The model under review builds one solid part; all positions refer to its coordinate system, in mm. A direction names the side the tool comes from. Coordinates: 2 decimals unless noted, no trailing zeros. Loops run counter-clockwise (first coordinate to the right, second up) from the corner with the lowest first, then second, coordinate; pieces in that order, holes last. Notation, with made-up numbers: M 13.25,-31.75 L 57.25,-31.75 A17 ccw 57.25,-21.75 Z; hole C 14.5,30 d11. An arc over 180 degrees is marked long. Return JSON: item names as keys, results as strings.
```python
from build123d import *

# Parameters (mm, degrees)
CROQUIS2_R              = 45
CROQUIS2_R_2            = 41
SALIENTE_EXTRUIR1_DEPTH = 10
CROQUIS3_R              = 45
SALIENTE_EXTRUIR2_DEPTH = 10
CROQUIS4_R              = 45
CROQUIS4_R_2            = 39.9
SALIENTE_EXTRUIR3_DEPTH = 3
CROQUIS5_R              = 2.5
CORTAR_EXTRUIR1_DEPTH   = 10


with BuildPart() as part:
    # Croquis2 → Saliente-Extruir1 (new body)
    with BuildSketch(Plane(origin=(0, 0, 0), x_dir=(0, 0, -1), z_dir=(1, 0, 0))):
        with Locations((-3.334066787, 2.439156595)):
            Circle(CROQUIS2_R)
        with Locations((-3.334066787, 2.439156595)):
            Circle(CROQUIS2_R_2, mode=Mode.SUBTRACT)
    extrude(amount=SALIENTE_EXTRUIR1_DEPTH)

    # Croquis3 → Saliente-Extruir2 (add)
    with BuildSketch(Plane(origin=(0, 0, 0), x_dir=(0, 0, -1), z_dir=(1, 0, 0))):
        with Locations((-3.334066787, 2.439156595)):
            Circle(CROQUIS3_R)
    extrude(amount=-SALIENTE_EXTRUIR2_DEPTH)

    # Croquis4 → Saliente-Extruir3 (add)
    with BuildSketch(Plane(origin=(10, 0, 0), x_dir=(0, 0, -1), z_dir=(1, 0, 0))):
        with Locations((-3.334066787, 2.439156595)):
            Circle(CROQUIS4_R)
        with Locations((-3.334066787, 2.439156595)):
            Circle(CROQUIS4_R_2, mode=Mode.SUBTRACT)
    extrude(amount=-SALIENTE_EXTRUIR3_DEPTH)

    # Croquis5 → Cortar-Extruir1 (cut)
    with BuildSketch(Plane(origin=(0, 0, 0), x_dir=(0, 0, -1), z_dir=(1, 0, 0))):
        with Locations((-3.334066787, 2.439156595)):
            Circle(CROQUIS5_R)
    extrude(amount=-CORTAR_EXTRUIR1_DEPTH, mode=Mode.SUBTRACT)


solid = part.part
```
1. Add section D-D on x = 1.75. Give the boundary of the cut face in (y, z).
Check values:
{"outline": "C 2.44,3.33 d90; hole C 2.44,3.33 d82"}
2. Add section B-B on y = -7. Give the boundary of the cut face in (x, z), plus the area to 3 significant figures.
Check values:
{"outline": "M -10,-40.66 L 10,-40.66 L 10,-35.43 L 7,-35.43 L 7,-36.56 L 0,-36.56 L 0,43.23 L 7,43.23 L 7,42.1 L 10,42.1 L 10,47.33 L -10,47.33 Z", "area": "969 mm²"}
3. Add section C-C on z = 2.5. Give the boundary of the cut face in (x, y), plus the area to 3 significant figures.
Check values:
{"outline": "M -10,-42.55 L 10,-42.55 L 10,-37.45 L 7,-37.45 L 7,-38.55 L 0,-38.55 L 0,0.08 L -10,0.08 Z; M -10,4.8 L 0,4.8 L 0,43.43 L 7,43.43 L 7,42.33 L 10,42.33 L 10,47.43 L -10,47.43 Z", "area": "939 mm²"}
4. Insertion check: pin 1 Ø1.5 at (x, z) = (-3, -17) entering from +Y; pin 2 Ø5 at (y, z) = (30.5, 5) entering from +X; pin 3 Ø10 at (x, z) = (-5, -12) entering from +Y; pin 4 Ø8 at (y, z) = (2.44, 3.33) entering from -X. Each pin has a flat end and moves straight along its axis. Give the tip position at first contact, or say it passes through.
Check values:
{"pin 1": "y = 42.95", "pin 2": "x = 0", "pin 3": "y = 46.24", "pin 4": "x = -10"}
5. The part is to be moulded in two halves that separate along X. For faces 1 (the face through (0.14, -41.49, 13.09)), 2 (the face through (3.451, -37.586, 12.222)), 3 (the face through (-10, 3, -6)), say which applies: released by +X, released by -X, zero draft, split by the parting line, or undercut.
Check values:
{"face 1": "zero draft", "face 2": "undercut", "face 3": "released by -X"}
6. Add section A-A on z = 27.5. Give the boundary of the cut face in (x, y).
Check values:
{"outline": "M -10,-35.52 L 10,-35.52 L 10,-29.31 L 7,-29.31 L 7,-30.68 L 0,-30.68 L 0,35.56 L 7,35.56 L 7,34.19 L 10,34.19 L 10,40.4 L -10,40.4 Z"}
7. Machinability: for faces 4 (the face through (7, -37, -6)), 5 (the face through (-4.93, 3.19, 0.95)), 6 (the face through (8.52, 36.08, -18.12)), which of the approach directions +Z, -Z, +X, -X, +Y, -Y give a long, thin tool a straight path to every point of the face, cutting with its end or side? Answer none if there is none.
Check values:
{"face 4": "none", "face 5": "+X, -X", "face 6": "+X"}
8. To check wall thickness, follow line 1 (X direction, y = 38, z = 15.5); line 2 (X direction, y = -25.5, z = 33); line 3 (Y direction, x = 3, z = -8). State the ranges of each line that lie inside material, in increasing order.
Check values:
{"line 1": "-10 to 0", "line 2": "-10 to 0, 7 to 10", "line 3": "-41.11 to -36.96, 41.84 to 45.99"}
